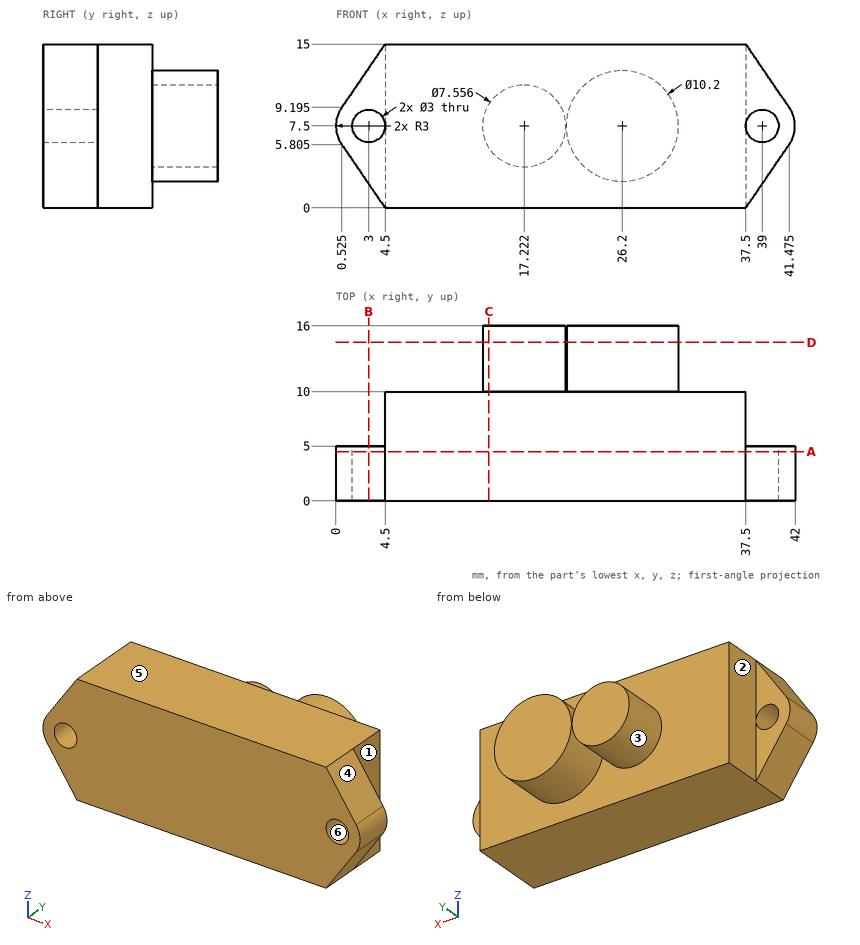
Job drawing, mm, ordinate dimensions from the low corner. One solid piece. A direction names the side the tool comes from. Coordinates: 2 decimals unless noted, no trailing zeros. Write each loop counter-clockwise with the first axis right and the second up, starting at its lowest first coordinate (ties: lowest second). Pieces come first, ordered by that corner, then holes. Notation, with made-up numbers: (50.25, 88.5) -> (77.25, 88.5) arc R15 cw to (77.25, 114.5) -> close; hole circle Ø10 at (74, 39). An arc over 180 degrees is marked (long way). Use CSV: the item, a comma, the result in double quotes. Start each with the question number.
Item 1: Band-saw the part on A-A, the plane y = 4.5. Write the cut outline in (x, z) (1 decimal), plus the area to 3 significant figures.
Item 2: Drop flat-ended pins along their axis: P1, Ø1.3, axis at x = 2.5, z = 10, coming from the +Y side; P2, Ø2, axis at y = 7.5, z = 12.5, coming from the -X side; P3, Ø1.5, axis at y = 8.5, z = 4.5, coming from the +X side. Give the stop position or say it passes through.
Item 3: Tool access for the marked faces 1, 2 and 3: list every direction of +Z, -Z, +X, -X, +Y, -Y with a clear straight run to the whole face (end or side of a thin tool).
Item 4: Band-saw the part on C-C, the plane x = 14. Write the cut outline in (y, z), plus the area to 3 significant figures.
Item 5: Band-saw the part on B-B, the plane x = 3. Write the cut outline in (y, z).
Item 6: Two-plate mould, pull along X, no slides. Class the marked faces 4, 5 and 6: +X half, -X half, draft (parallel to the pull), parting line (faces both ways), or undercut.
Item 7: Band-saw the part on D-D, the plane y = 14.5. Write the cut outline in (x, z).
Item 8: Wall check: probe 1 along X at (y, z) = (2.5, 7.5); probe 2 along Y at (x, z) = (12, 14.5); probe 3 along X at (y, z) = (7, 5.75). Give the ranges that are in metal, low to high.
Response values:
1,outline,"(0.5, 5.8) -> (4.5, 0) -> (37.5, 0) -> (41.5, 5.8) arc R3 ccw to (41.5, 9.2) -> (37.5, 15) -> (4.5, 15) -> (0.5, 9.2) arc R3 ccw to start; hole circle Ø3 at (3, 7.5); hole circle Ø3 at (39, 7.5)"
1,area,"556 mm2"
2,P1,"stops at y = 5"
2,P2,"stops at x = 4.5"
2,P3,"stops at x = 37.5"
3,face 1,"+Z, -Z, +X, +Y"
3,face 2,"+Z, -Z, -X, +Y"
3,face 3,"+Y"
4,outline,"(0, 0) -> (10, 0) -> (10, 5.53) -> (16, 5.53) -> (16, 9.47) -> (10, 9.47) -> (10, 15) -> (0, 15) -> close"
4,area,"174 mm2"
5,outline,"(0, 2.19) -> (5, 2.19) -> (5, 6) -> (0, 6) -> close; (0, 9) -> (5, 9) -> (5, 12.81) -> (0, 12.81) -> close"
6,face 4,"+X half"
6,face 5,"draft"
6,face 6,"undercut"
7,outline,"circle Ø7.56 at (17.22, 7.5); circle Ø10.2 at (26.2, 7.5)"
8,probe 1,"x = 0 to 1.5, 4.5 to 37.5, 40.5 to 42"
8,probe 2,"y = 0 to 10"
8,probe 3,"x = 4.5 to 37.5"
